Check sheet for the modelled part. Datum: model origin and axes. Units: mm. A direction names the side the tool comes from. Round coordinates to 2 decimals unless told otherwise and drop trailing zeros. Write each loop counter-clockwise with the first axis right and the second up, starting at its lowest first coordinate (ties: lowest second). Pieces come first, ordered by that corner, then holes. Notation, with made-up numbers: M 19.5,34 L 34.5,34 A26 cw 34.5,56 Z; hole C 27.25,-32.75 d9. An arc over 180 degrees is marked long. Answer in a Markdown table with one row per item.
```python
from build123d import *

# Parameters (mm, degrees)
SKETCH_1_W          = 30
SKETCH_1_H          = 38
EXTRUDE_1_DEPTH     = 3
SKETCH_2_W          = 30
SKETCH_2_H          = 3
EXTRUDE_2_DEPTH     = 35
SKETCH_3_R          = 1.5
CUT_EXTRUDE_1_DEPTH = 35
SKETCH_4_R          = 1.5
CUT_EXTRUDE_2_DEPTH = 35
SKETCH_5_W          = 88.636762999
SKETCH_5_H          = 63.593874591
CUT_EXTRUDE_3_DEPTH = 1
SKETCH_6_W          = 48.892654417
SKETCH_6_H          = 42.932057718
CUT_EXTRUDE_4_DEPTH = 1
SKETCH_7_W          = 36.310850366
SKETCH_7_H          = 6.739338697
CUT_EXTRUDE_5_DEPTH = 7
SKETCH_8_W          = 38.639290764
SKETCH_8_H          = 12.957782525
CUT_EXTRUDE_6_DEPTH = 17


with BuildPart() as part:
    # 草图1 → 凸台-拉伸1 (new body)
    with BuildSketch(Plane.XY):
        Rectangle(SKETCH_1_W, SKETCH_1_H)
    extrude(amount=EXTRUDE_1_DEPTH)

    # 草图2 → 凸台-拉伸2 (add)
    with BuildSketch(Plane.XY.offset(3)):
        with Locations((0, -17.5)):
            Rectangle(SKETCH_2_W, SKETCH_2_H)
    extrude(amount=EXTRUDE_2_DEPTH)

    # 草图3 → 切除-拉伸1 (cut)
    with BuildSketch(Plane.XY.offset(3)):
        with Locations((-10, -6)):
            Circle(SKETCH_3_R)
        with Locations((10, -6)):
            Circle(SKETCH_3_R)
    extrude(amount=-CUT_EXTRUDE_1_DEPTH, mode=Mode.SUBTRACT)

    # 草图4 → 切除-拉伸2 (cut)
    with BuildSketch(Plane(origin=(0, -16, 0), x_dir=(1, 0, 0), z_dir=(0, 1, 0))):
        with Locations((-10, -23)):
            Circle(SKETCH_4_R)
        with Locations((10, -23)):
            Circle(SKETCH_4_R)
    extrude(amount=-CUT_EXTRUDE_2_DEPTH, mode=Mode.SUBTRACT)

    # 草图5 → 切除-拉伸3 (cut)
    with BuildSketch(Plane.XZ.offset(19)):
        with Locations((3.130084419, 17.677441591)):
            Rectangle(SKETCH_5_W, SKETCH_5_H)
    extrude(amount=-CUT_EXTRUDE_3_DEPTH, mode=Mode.SUBTRACT)

    # 草图6 → 切除-拉伸4 (cut)
    with BuildSketch(Plane(origin=(0, 0, 0), x_dir=(-1, 0, 0), z_dir=(0, 0, -1))):
        with Locations((1.260467489, 1.250792639)):
            Rectangle(SKETCH_6_W, SKETCH_6_H)
    extrude(amount=-CUT_EXTRUDE_4_DEPTH, mode=Mode.SUBTRACT)

    # 草图7 → 切除-拉伸5 (cut)
    with BuildSketch(Plane.XY.offset(38)):
        with Locations((-0.942459464, -16.150780979)):
            Rectangle(SKETCH_7_W, SKETCH_7_H)
    extrude(amount=-CUT_EXTRUDE_5_DEPTH, mode=Mode.SUBTRACT)

    # 草图8 → 切除-拉伸6 (cut)
    with BuildSketch(Plane(origin=(0, 19, 0), x_dir=(1, 0, 0), z_dir=(0, 1, 0))):
        with Locations((-0.082193205, -0.869277183)):
            Rectangle(SKETCH_8_W, SKETCH_8_H)
    extrude(amount=-CUT_EXTRUDE_6_DEPTH, mode=Mode.SUBTRACT)


solid = part.part
```
1. Access from +Z, -Z, +X, -X, +Y, -Y to the whole of each face (thin tool, end or side, straight path). Record for faces 1 (the face through (-11.5, -5.93, 2.01)), 2 (the face through (0, -7, 3)).
Found:
| item | result |
|---|---|
| face 1 | +Z, -Z |
| face 2 | +Z, +X, -X, +Y |
2. Section check D-D, the plane y = -16.5. Record the cut outline in (x, z).
Found:
| item | result |
|---|---|
| outline | M -15,1 L 15,1 L 15,31 L -15,31 Z; hole C -10,23 d3; hole C 10,23 d3 |
3. Section check C-C, the plane y = -6. Record the cut outline in (x, z), and give its area (3 significant figures).
Found:
| item | result |
|---|---|
| outline | M -15,1 L -11.5,1 L -11.5,3 L -15,3 Z; M -8.5,1 L 8.5,1 L 8.5,3 L -8.5,3 Z; M 11.5,1 L 15,1 L 15,3 L 11.5,3 Z |
| area | 48.0 mm2 |
4. Section check A-A, the plane z = 23. Record the cut outline in (x, y).
Found:
| item | result |
|---|---|
| outline | M -15,-18 L -11.5,-18 L -11.5,-16 L -15,-16 Z; M -8.5,-18 L 8.5,-18 L 8.5,-16 L -8.5,-16 Z; M 11.5,-18 L 15,-18 L 15,-16 L 11.5,-16 Z |
5. Go/stop test with flat-tipped pins: pin 1 (2 mm diameter, centred on x = -3.5, y = -4.5, fed in from +Z); pin 2 (5 mm diameter, centred on x = 11, z = 17, fed in from +Y); pin 3 (2.5 mm diameter, centred on x = -10, z = 23, fed in from +Y). Record where each tip stops, or that it passes through.
Found:
| item | result |
|---|---|
| pin 1 | stops at z = 3 |
| pin 2 | stops at y = -16 |
| pin 3 | passes through |
6. Section check B-B, the plane x = 10. Record the cut outline in (y, z), and give its area (3 significant figures).
Found:
| item | result |
|---|---|
| outline | M -18,1 L -7.5,1 L -7.5,3 L -16,3 L -16,21.5 L -18,21.5 Z; M -18,24.5 L -16,24.5 L -16,31 L -18,31 Z; M -4.5,1 L 2,1 L 2,3 L -4.5,3 Z |
| area | 84.0 mm2 |
7. Scan lines: L1, parallel to X at y = -16.4, z = 23; L2, parallel to Y at x = 10, z = 2.5; L3, parallel to Z at x = -10, y = -17.6. Record each from-to range of solid material in increasing order.
Found:
| item | result |
|---|---|
| L1 | x = -15 to -11.5, -8.5 to 8.5, 11.5 to 15 |
| L2 | y = -18 to -7.5, -4.5 to 2 |
| L3 | z = 1 to 21.5, 24.5 to 31 |
8. Draft check along Y on faces 3 (the face through (0, -16, 17)), 4 (the face through (8.5, -5.93, 2.01)), 5 (the face through (0, -8, 1)). Enter one of: +Y half, -Y half, draft (parallel to the pull), parting line (faces both ways), or undercut.
Found:
| item | result |
|---|---|
| face 3 | +Y half |
| face 4 | undercut |
| face 5 | draft |
